Read the model definition and answer for the solid it produces. Units are mm, in the model's axes. A direction names the side the tool comes from. Give positions to 0.01 mm unless a question says otherwise; leave off trailing zeros. Order: outer loops, then holes, each group sorted by start corner. A loop starts at its lowest first (then second) coordinate and runs counter-clockwise, first axis right, second up. Notation, with made-up numbers: (6.5, 79) - (59.5, 79) arc R27 cw to (59.5, 105) - close; hole circle Ø11 at (81, 59.25). An arc over 180 degrees is marked (long way). Write each question's results on one line, items separated by ' | '. Start each with the question number.
Q1. A tool of negligible diameter and unlimited length cuts with its end or side. For faces 1 (the face through (-26.34, -4.6, -54.52)), 2 (the face through (-1.214, -8.354, -52.682)), from which of +Z, -Z, +X, -X, +Y, -Y can it reach the whole face along a straight path? Write none if from no direction.
Q2. Find section A-A on x = 0. Give the vertices of the cut face in (y, z) (3 decimals).
Q3. Find the intervals of material crossed by line 1 along Z through (x, y) = (0, -8.7) (3 decimals); line 2 along Z through (x, y) = (1, -7.75) (3 decimals); line 3 along Z through (x, y) = (21, -3.25), in increasing order. Write a range as from..to.
Q4. A flat-ended cylindrical pin translates along its axis: P1, Ø2.5, axis at x = -9.5, z = 47.5, coming from the -Y side. Find the tip coordinate at first contact, or state that the pin passes through.
from build123d import *

# Parameters (mm, degrees)
F1_DEPTH = 9.34
F2_R     = 2.4
F2_R_2   = 5.6
F3_DEPTH = 2


with BuildPart() as f1:
    # F0 (on Front) → F1 (new body)
    with BuildSketch(Plane.XZ):
        with BuildLine():
            ThreePointArc((28.675, 48.7962), (26.279485, 54.579485), (20.4962, 56.975))
            Line((20.4962, 56.975), (-20.4962, 56.975))
            ThreePointArc((-20.4962, 56.975), (-26.279485, 54.579485), (-28.675, 48.7962))
            Line((-28.675, 48.7962), (-28.675, -48.7962))
            ThreePointArc((-28.675, -48.7962), (-26.279485, -54.579485), (-20.4962, -56.975))
            Line((-20.4962, -56.975), (20.4962, -56.975))
            ThreePointArc((20.4962, -56.975), (26.279485, -54.579485), (28.675, -48.7962))
            Line((28.675, -48.7962), (28.675, 48.7962))
        make_face()
    extrude(amount=F1_DEPTH)

    # F2 (on face) → F3 (cut)
    with BuildSketch(Plane.XZ.offset(9.34)):
        with Locations((-9.405, 46.685)):
            Circle(F2_R)
        with BuildLine():
            Line((-4.25, 45.335), (4.25, 45.335))
            ThreePointArc((4.25, 45.335), (5.204594, 45.730406), (5.6, 46.685))
            ThreePointArc((5.6, 46.685), (5.204594, 47.639594), (4.25, 48.035))
            Line((4.25, 48.035), (-4.25, 48.035))
            ThreePointArc((-4.25, 48.035), (-5.204594, 47.639594), (-5.6, 46.685))
            ThreePointArc((-5.6, 46.685), (-5.204594, 45.730406), (-4.25, 45.335))
        make_face()
        with Locations((0, -47.215)):
            Circle(F2_R_2)
    extrude(amount=-F3_DEPTH, mode=Mode.SUBTRACT)


solid = f1.part
Working result:
1) face 1: -Z, -X, +Y, -Y | face 2: -Y
2) outline: (-9.34, -56.975) - (0, -56.975) - (0, 56.975) - (-9.34, 56.975) - (-9.34, 48.035) - (-7.34, 48.035) - (-7.34, 45.335) - (-9.34, 45.335) - (-9.34, -41.615) - (-7.34, -41.615) - (-7.34, -52.815) - (-9.34, -52.815) - close
3) line 1: -56.975..-52.815, -41.615..45.335, 48.035..56.975 | line 2: -56.975..-52.725, -41.705..45.335, 48.035..56.975 | line 3: -56.96..56.96
4) P1: y = -7.34
